from build123d import *

# Parameters (mm, degrees)
F1_DEPTH     = 9
F2_T1_DEPTH  = 21.5
F2_T3_DEPTH  = 99
F2_T6_ANGLE  = 90
F2_T8_ANGLE  = 90
F2_T10_ANGLE = 90
F2_T12_ANGLE = 90
F3_R         = 1.75
F4_DEPTH     = 13


# Not quite as in the source:
# - a fillet or chamfer that OpenCascade refuses, or shapes differently, is made with other operations: its cross-section is extruded or revolved along the edge and cut away or added


with BuildPart() as f1:
    # F0 (on Top) → F1 (new body)
    with BuildSketch(Plane.XY):
        with BuildLine():
            Line((0, 9), (0, 0))
            Line((0, 0), (9, 0))
            Line((9, 0), (9, 9))
            ThreePointArc((9, 9), (11.9289321881, 16.0710678119), (19, 19))
            Line((19, 19), (118, 19))
            ThreePointArc((118, 19), (125.0710678119, 16.0710678119), (128, 9))
            Line((128, 9), (128, 0))
            Line((128, 0), (137, 0))
            Line((137, 0), (137, 9))
            ThreePointArc((137, 9), (131.4350288425, 22.4350288425), (118, 28))
            Line((118, 28), (19, 28))
            ThreePointArc((19, 28), (5.5649711575, 22.4350288425), (0, 9))
        make_face()
    extrude(amount=F1_DEPTH)

    # F2: fillet of radius 5 on 7 edges, made by hand

    # F2_s2 → F2_t1 (cut)
    with BuildSketch(Plane.XZ.offset(-9)):
        with BuildLine():
            ThreePointArc((0, 4), (1.4644660941, 7.5355339059), (5, 9))
            Line((5, 9), (0, 9))
            Line((0, 9), (0, 4))
        make_face()
        with BuildLine():
            ThreePointArc((137, 4), (135.5355339059, 7.5355339059), (132, 9))
            Line((132, 9), (137, 9))
            Line((137, 9), (137, 4))
        make_face()
        with BuildLine():
            ThreePointArc((128, 4), (129.4644660941, 7.5355339059), (133, 9))
            Line((133, 9), (128, 9))
            Line((128, 9), (128, 4))
        make_face()
        with BuildLine():
            ThreePointArc((9, 4), (7.5355339059, 7.5355339059), (4, 9))
            Line((4, 9), (9, 9))
            Line((9, 9), (9, 4))
        make_face()
    extrude(amount=F2_T1_DEPTH, mode=Mode.SUBTRACT)

    # F2_s4 → F2_t3 (cut)
    with BuildSketch(Plane.YZ.offset(19)):
        with BuildLine():
            ThreePointArc((28, 4), (26.5355339059, 7.5355339059), (23, 9))
            Line((23, 9), (28, 9))
            Line((28, 9), (28, 4))
        make_face()
        with BuildLine():
            ThreePointArc((19, 4), (20.4644660941, 7.5355339059), (24, 9))
            Line((24, 9), (19, 9))
            Line((19, 9), (19, 4))
        make_face()
    extrude(amount=F2_T3_DEPTH, mode=Mode.SUBTRACT)

    # F2_s5 → F2_t6 (revolve, cut)
    with BuildSketch(Plane.YZ.offset(19)):
        with BuildLine():
            ThreePointArc((28, 4), (26.5355339059, 7.5355339059), (23, 9))
            Line((23, 9), (28, 9))
            Line((28, 9), (28, 4))
        make_face()
    revolve(axis=Axis((19, 9, 9), (0, 0, 1)), revolution_arc=F2_T6_ANGLE, mode=Mode.SUBTRACT)

    # F2_s7 → F2_t8 (revolve, cut)
    with BuildSketch(Plane.XZ.offset(-9)):
        with BuildLine():
            ThreePointArc((137, 4), (135.5355339059, 7.5355339059), (132, 9))
            Line((132, 9), (137, 9))
            Line((137, 9), (137, 4))
        make_face()
    revolve(axis=Axis((118, 9, 9), (0, 0, 1)), revolution_arc=F2_T8_ANGLE, mode=Mode.SUBTRACT)

    # F2_s9 → F2_t10 (revolve, cut)
    with BuildSketch(Plane.YZ.offset(118)):
        with BuildLine():
            ThreePointArc((19, 4), (20.4644660941, 7.5355339059), (24, 9))
            Line((24, 9), (19, 9))
            Line((19, 9), (19, 4))
        make_face()
    revolve(axis=Axis((118, 9, 9), (0, 0, -1)), revolution_arc=F2_T10_ANGLE, mode=Mode.SUBTRACT)

    # F2_s11 → F2_t12 (revolve, cut)
    with BuildSketch(Plane.XZ.offset(-9)):
        with BuildLine():
            ThreePointArc((9, 4), (7.5355339059, 7.5355339059), (4, 9))
            Line((4, 9), (9, 9))
            Line((9, 9), (9, 4))
        make_face()
    revolve(axis=Axis((19, 9, 9), (0, 0, -1)), revolution_arc=F2_T12_ANGLE, mode=Mode.SUBTRACT)

    # F3 (on face) → F4 (cut)
    with BuildSketch(Plane.XZ):
        with Locations((4.5, 4.5)):
            Circle(F3_R)
        with Locations((132.5, 4.5)):
            Circle(F3_R)
    extrude(amount=-F4_DEPTH, mode=Mode.SUBTRACT)


solid = f1.part
Verification items for the finished model (mm, model axes). A direction names the side the tool comes from. Coordinates: 2 decimals unless noted, no trailing zeros. Write each loop counter-clockwise with the first axis right and the second up, starting at its lowest first coordinate (ties: lowest second). Pieces come first, ordered by that corner, then holes. Notation, with made-up numbers: (20.25, 38) -> (25.25, 38) arc R12 cw to (25.25, 51) -> close; hole circle Ø7 at (1, 71). An arc over 180 degrees is marked (long way). One line per item, written item: value. Start each with the question number.
Q1. Access from +Z, -Z, +X, -X, +Y, -Y to the whole of each face (thin tool, end or side, straight path). Record for faces 1 (the cylindrical face through (134.169, 6.409, 5.026)), 2 (the cylindrical face through (129, 5, 7)), 3 (the cylindrical face through (11.85, 15.99, 1.97)), 4 (the flat face through (69, 28, 2)).
Q2. Go/stop test with flat-tipped pins: P1, Ø1.8, axis at x = 132, z = 4.5, coming from the -Y side; P2, Ø2, axis at y = 20, z = 4, coming from the +X side; P3, Ø1, axis at x = 122, z = 5.5, coming from the -Y side; P4, Ø12, axis at x = 102.5, y = 8.5, coming from the +Z side. Record where each tip stops, or that it passes through.
Q3. Cross-section at C-C on x = 25. Enter the section's corners in (y, z).
Q4. Mould release check, pull along X, two halves, no side actions. Record for faces 5 (the flat face through (128, 5, 2)), 6 (the flat face through (0, 5, 2)), 7 (the flat face through (68, 20, 0)): pulls with the +X half, pulls with the -X half, needs draft (parallel to the pull), parting line crosses it, or undercut.
Q5. Cross-section at A-A on y = 5.25. Enter the section's corners in (x, z), and give its area (3 significant figures).
Q6. Thickness scan on L1, parallel to X at y = 2.5, z = 2.5; L2, parallel to Z at x = 4.5, y = 4; L3, parallel to X at y = 8, z = 4. Record the ranges inside material, lowest first. Write a range as from..to.
Q7. Cross-section at B-B on z = 1.5. Enter the section's corners in (x, y), and give its area (3 significant figures).
Checked values:
1. face 1: -Y
1. face 2: +Z, -Y
1. face 3: +Z, -Z, -Y
1. face 4: +Z, -Z, +X, -X, +Y
2. P1: stops at y = 13
2. P2: stops at x = 134.16
2. P3: stops at y = 18.14
2. P4: passes through
3. outline: (19, 0) -> (28, 0) -> (28, 4) arc R5 ccw to (23.5, 8.97) arc R5 ccw to (19, 4) -> close
4. face 5: undercut
4. face 6: pulls with the -X half
4. face 7: needs draft
5. outline: (0, 0) -> (9, 0) -> (9, 4) arc R5 ccw to (4.5, 8.97) arc R5 ccw to (0, 4) -> close; (128, 0) -> (137, 0) -> (137, 4) arc R5 ccw to (132.5, 8.97) arc R5 ccw to (128, 4) -> close; hole circle Ø3.5 at (4.5, 4.5); hole circle Ø3.5 at (132.5, 4.5)
5. area: 121 mm²
6. L1: x = 0..9, 128..137
6. L2: z = 0..2.75, 6.25..8.97
6. L3: x = 0..2.82, 6.18..9, 128..130.82, 134.18..137
7. outline: (0, 0) -> (9, 0) -> (9, 9) arc R10 cw to (19, 19) -> (118, 19) arc R10 cw to (128, 9) -> (128, 0) -> (137, 0) -> (137, 9) arc R19 ccw to (118, 28) -> (19, 28) arc R19 ccw to (0, 9) -> close
7. area: 1,460 mm²
